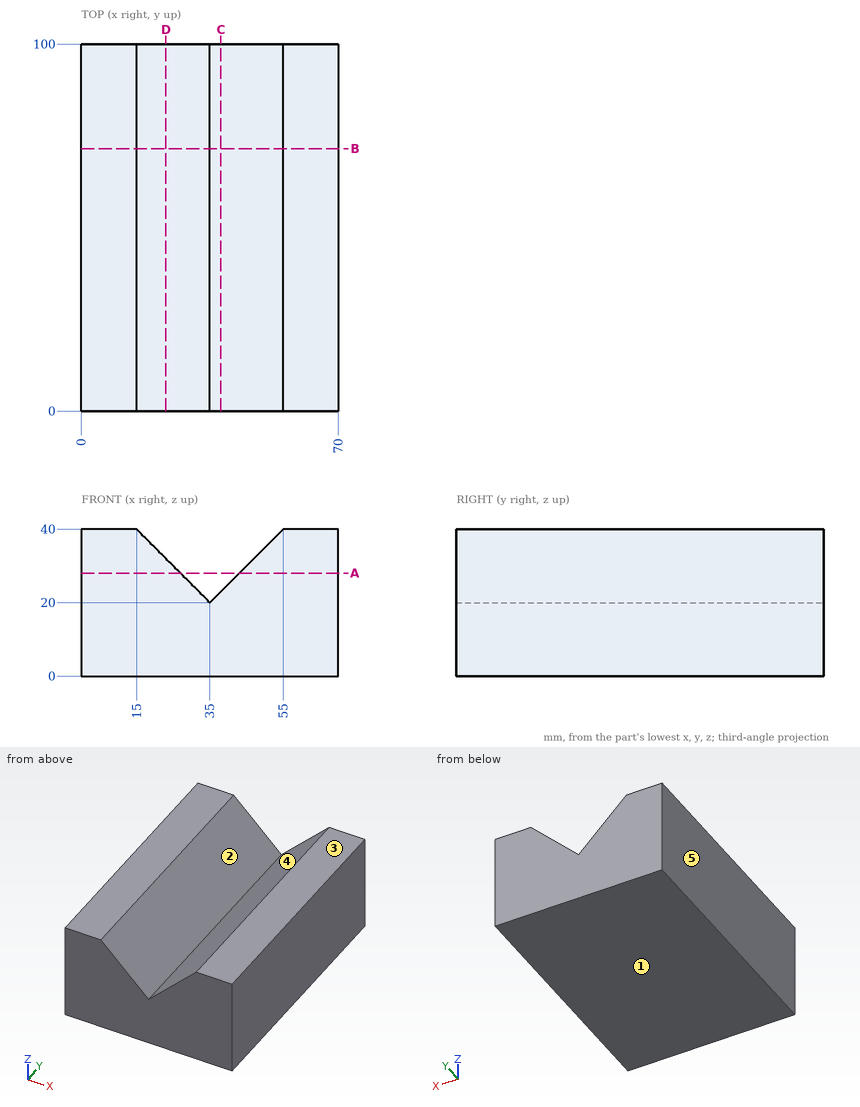
Check sheet for the drawn part. Datum: minimum x, y, z corner. Units: mm. A direction names the side the tool comes from. Round coordinates to 2 decimals unless told otherwise and drop trailing zeros. Order: outer loops, then holes, each group sorted by start corner. A loop starts at its lowest first (then second) coordinate and runs counter-clockwise, first axis right, second up. Notation, with made-up numbers: (39, 6) -> (88, 6) arc R17 cw to (88, 16) -> close; hole circle Ø4 at (8.25, 68). An arc over 180 degrees is marked (long way). Use CSV: the item, a comma, the result in double quotes.
(1) Depth check by flat-ended pin: pin 1 (3 mm diameter, centred on x = 50, z = 9.5, fed in from -Y); pin 2 (5 mm diameter, centred on x = 24, y = 89, fed in from +Z); pin 3 (6 mm diameter, centred on x = 26, y = 20, fed in from +Z). Enter the tip coordinate at first touch or a pass-through.
Worked out:
pin 1,"y = 0"
pin 2,"z = 33.5"
pin 3,"z = 32"
(2) Material ranges on line 1 along X through (y, z) = (61, 22); line 2 along X through (y, z) = (34, 37); line 3 along Z through (x, y) = (40, 82), recorded low to high. Write a range as from..to.
Worked out:
line 1,"0..33, 37..70"
line 2,"0..18, 52..70"
line 3,"0..25"
(3) Cross-section at C-C (x = 38). Record the boundary of the cut face in (y, z).
Worked out:
outline,"(0, 0) -> (100, 0) -> (100, 23) -> (0, 23) -> close"
(4) Cross-section at B-B (y = 71.5). Record the boundary of the cut face in (x, z), and give its area (3 significant figures).
Worked out:
outline,"(0, 0) -> (70, 0) -> (70, 40) -> (55, 40) -> (35, 20) -> (15, 40) -> (0, 40) -> close"
area,"2,400 mm²"
(5) Cross-section at D-D (x = 23). Record the boundary of the cut face in (y, z).
Worked out:
outline,"(0, 0) -> (100, 0) -> (100, 32) -> (0, 32) -> close"
(6) Cross-section at A-A (z = 28). Record the boundary of the cut face in (x, y).
Worked out:
outline,"(0, 0) -> (27, 0) -> (27, 100) -> (0, 100) -> close; (43, 0) -> (70, 0) -> (70, 100) -> (43, 100) -> close"
(7) Tool access check on the marked faces 1 and 2. Record the directions out of +Z, -Z, +X, -X, +Y, -Y that give a thin tool (end or side, any length) a straight path to the whole face; none if there is none.
Worked out:
face 1,"-Z, +X, -X, +Y, -Y"
face 2,"+Z, +Y, -Y"
(8) Draft check along X on the marked faces 3, 4 and 5. Enter one of: pulls with the +X half, pulls with the -X half, needs draft (parallel to the pull), parting line crosses it, or undercut.
Worked out:
face 3,"needs draft"
face 4,"undercut"
face 5,"pulls with the -X half"
